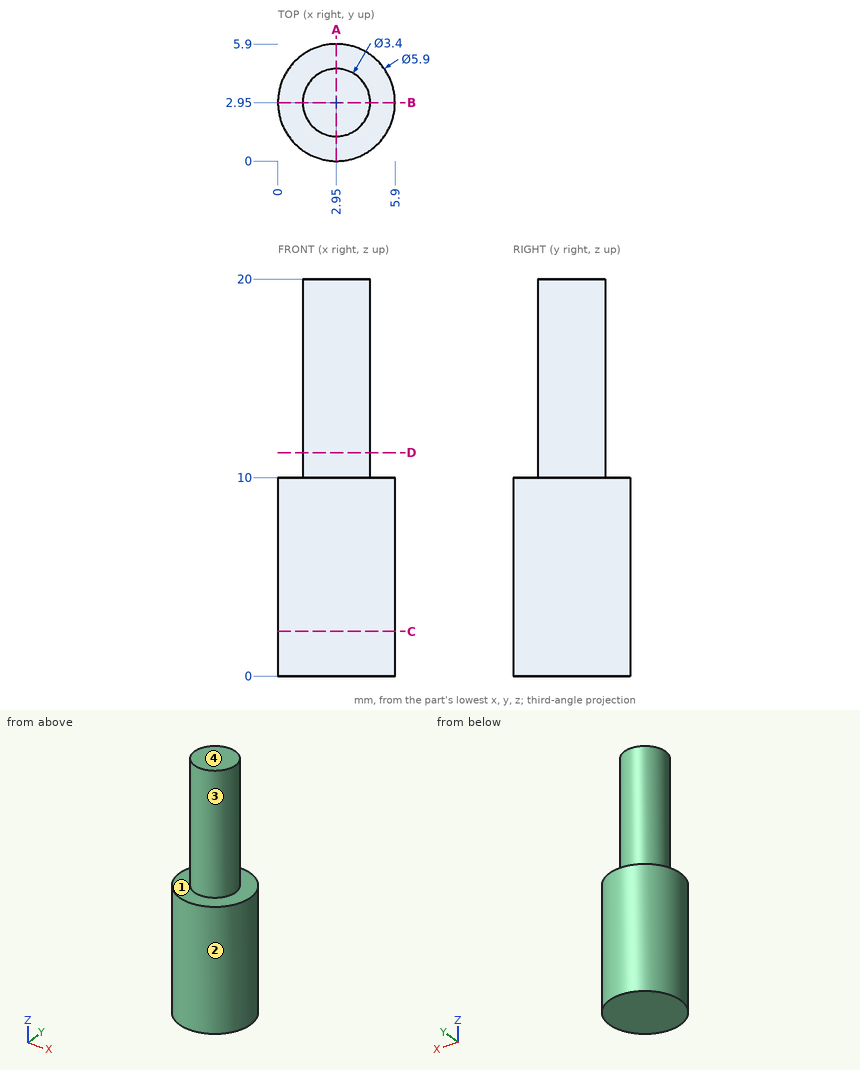
Input: dimensioned drawing with shaded views. Units: mm. Origin: part minimum x, y, z. A direction names the side the tool comes from. Coordinates: 2 decimals unless noted, no trailing zeros. Order: outer loops, then holes, each group sorted by start corner. A loop starts at its lowest first (then second) coordinate and runs counter-clockwise, first axis right, second up. Notation, with made-up numbers: M 67,34.5 L 110,34.5 A22 ccw 110,48.5 Z; hole C 84.5,-24 d6. An arc over 180 degrees is marked long. Write each question's results on one line, items separated by ' | '. Start each with the question number.
Item 1: Cut plane D-D (z = 11.25). Return loops of the section in (x, y).
Item 2: First-contact query: pin 1 Ø1 at (y, z) = (3.5, 17.5) entering from -X; pin 2 Ø1 at (y, z) = (0.5, 13.5) entering from +X. Flat tips, straight axial feed; report the tip coordinate or a pass-through.
Item 3: Line query: probe 1 along Y at (x, z) = (3.05, 6.5); probe 2 along Z at (x, y) = (3.6, 4.8); probe 3 along Y at (x, z) = (2.5, 12). Output: solid intervals per line, ascending.
Item 4: Cut plane A-A (x = 2.95). Return loops of the section in (y, z), and give its area (3 significant figures).
Item 5: Set-up query: the marked faces 1 and 2. Return all of +Z, -Z, +X, -X, +Y, -Y with unobstructed straight access to the full face (end or side cutting, diameter ignored); none if empty.
Item 6: Cut plane C-C (z = 2.25). Return loops of the section in (x, y).
Item 7: Draft query along X for the marked faces 3 and 4. Return one class per face: pulls with the +X half, pulls with the -X half, needs draft (parallel to the pull), parting line crosses it, or undercut.
Checked values:
1) outline: C 2.95,2.95 d3.4
2) pin 1: stops at x = 1.25 | pin 2: passes through
3) probe 1: y = 0 to 5.9 | probe 2: z = 0 to 10 | probe 3: y = 1.31 to 4.59
4) outline: M 0,0 L 5.9,0 L 5.9,10 L 4.65,10 L 4.65,20 L 1.25,20 L 1.25,10 L 0,10 Z | area: 93.0 mm2
5) face 1: +Z | face 2: +Z, -Z
6) outline: C 2.95,2.95 d5.9
7) face 3: parting line crosses it | face 4: needs draft
